```python
from build123d import *

# Parameters (mm, degrees)
BOSS_EXTRUDE1_DEPTH   = 20
BOSS_EXTRUDE1_2_DEPTH = 20
BOSS_EXTRUDE1_3_DEPTH = 20
BOSS_EXTRUDE1_4_DEPTH = 20
SKETCH2_W             = 20
SKETCH2_H             = 20
BOSS_EXTRUDE2_DEPTH   = 20
CUT_EXTRUDE1_DEPTH    = 31
BOSS_EXTRUDE3_DEPTH   = 30
FILLET1_R             = 7
CUT_EXTRUDE2_REACH    = 47.826
SKETCH5_R             = 2.7
CUT_EXTRUDE3_REACH    = 48.5
SKETCH6_R             = 5
FILLET5_R             = 1
FILLET6_R             = 0.75
CUT_EXTRUDE4_DEPTH    = 10


# Some blends are built 0.0001 mm under size
with BuildPart() as part:
    # Sketch1 → Boss-Extrude1 (new body)
    with BuildSketch(Plane(origin=(0, 0, 0), x_dir=(1, 0, 0), z_dir=(0, 1, 0))):
        Polygon((-10, -2.8), (-10, 2.8), (-7.7, 2.8), (-7.7, 5.58), (-7.135634919, 5.58), (-4.28, 2.724365081), (-4.28, -2.724365081), (-7.135634919, -5.58), (-7.7, -5.58), (-7.7, -2.8), align=None)
    extrude(amount=BOSS_EXTRUDE1_DEPTH)



with BuildPart() as body_2:
    # Sketch1 → Boss-Extrude1 2 (new body)
    with BuildSketch(Plane(origin=(0, 0, 0), x_dir=(1, 0, 0), z_dir=(0, 1, 0))):
        Polygon((10, 2.8), (7.7, 2.8), (7.7, 5.58), (7.135634919, 5.58), (4.28, 2.724365081), (4.28, -2.724365081), (7.135634919, -5.58), (7.7, -5.58), (7.7, -2.8), (10, -2.8), align=None)
    extrude(amount=BOSS_EXTRUDE1_2_DEPTH)


with BuildPart() as body_3:
    # Sketch1 → Boss-Extrude1 3 (new body)
    with BuildSketch(Plane(origin=(0, 0, 0), x_dir=(1, 0, 0), z_dir=(0, 1, 0))):
        Polygon((2.8, -10), (-2.8, -10), (-2.8, -7.7), (-5.58, -7.7), (-5.58, -7.135634919), (-2.724365081, -4.28), (2.724365081, -4.28), (5.58, -7.135634919), (5.58, -7.7), (2.8, -7.7), align=None)
    extrude(amount=BOSS_EXTRUDE1_3_DEPTH)


with BuildPart() as body_4:
    # Sketch1 → Boss-Extrude1 4 (new body)
    with BuildSketch(Plane(origin=(0, 0, 0), x_dir=(1, 0, 0), z_dir=(0, 1, 0))):
        Polygon((-2.8, 10), (-2.8, 7.7), (-5.58, 7.7), (-5.58, 7.135634919), (-2.724365081, 4.28), (2.724365081, 4.28), (5.58, 7.135634919), (5.58, 7.7), (2.8, 7.7), (2.8, 10), align=None)
    extrude(amount=BOSS_EXTRUDE1_4_DEPTH)


with BuildPart() as part_1:
    add(part.part)

    add(body_2.part)  # Boss-Extrude2 merges body 2

    add(body_3.part)  # Boss-Extrude2 merges body 3

    add(body_4.part)  # Boss-Extrude2 merges body 4
    # Sketch2 → Boss-Extrude2 (add)
    with BuildSketch(Plane.XZ):
        Rectangle(SKETCH2_W, SKETCH2_H)
    extrude(amount=BOSS_EXTRUDE2_DEPTH)

    # Sketch3 → Cut-Extrude1 (cut, through all)
    with BuildSketch(Plane(origin=(10, 0, 0), x_dir=(0, 0, -1), z_dir=(1, 0, 0))):
        Polygon((10.596673941, -8.137212268), (10.596673941, -38.345549702), (-10.411138478, -38.345549702), (-10.411138478, -2.402671747), align=None)
    extrude(amount=-CUT_EXTRUDE1_DEPTH, mode=Mode.SUBTRACT)

    # Sketch4 → Boss-Extrude3 (add)
    with BuildSketch(Plane.ZY.offset(10)):
        Polygon((10, 0), (-10, 0), (-10, -7.974337104), (10, -2.51490096), align=None)
    extrude(amount=BOSS_EXTRUDE3_DEPTH)

    # Fillet1
    # the kernel refuses this fillet: 7 mm, written as the material it takes off along each edge
    with BuildSketch(Plane(origin=(10, 2.093496024, 26.882318479), x_dir=(0, 0.9647039130954435, -0.26333697054978655), z_dir=(0, -0.26333697054978655, -0.9647039130954435))) as fillet1_piece_1:
        with BuildLine():
            CenterArc((FILLET1_R, -FILLET1_R), FILLET1_R, 90, 90)
            Line((0, -FILLET1_R), (0, 0))
            Line((0, 0), (FILLET1_R, 0))
        make_face()
    extrude(amount=55.731749637, mode=Mode.SUBTRACT)

    # Cut-Extrude2: up to this plane
    cut_extrude2_end = Plane(origin=(-10, -8.137212268, -10.596673941), z_dir=(0, 0.9647039130954435, -0.26333697054978655))
    # Sketch5 → Cut-Extrude2 (cut, up to the surface)
    with BuildSketch(Plane(origin=(0, 0, 0), x_dir=(1, 0, 0), z_dir=(0, 1, 0)), mode=Mode.PRIVATE) as cut_extrude2_sk1:
        with Locations(Location((-28.5, 0, 0), (0, 0, 270))):
            Circle(SKETCH5_R)
    cut_extrude2_tool1 = split(extrude(cut_extrude2_sk1.sketch, amount=-CUT_EXTRUDE2_REACH, mode=Mode.PRIVATE), bisect_by=cut_extrude2_end, keep=Keep.BOTH, mode=Mode.PRIVATE)
    add(cut_extrude2_tool1.solids().sort_by_distance((-28.5, 0, 0))[0], mode=Mode.SUBTRACT)

    # Cut-Extrude3: up to this plane
    cut_extrude3_end = Plane(origin=(-10, -8.137212268, -10.596673941), z_dir=(0, 0.9647039130954435, -0.26333697054978655))
    # Sketch6 → Cut-Extrude3 (cut, up to the surface)
    with BuildSketch(Plane(origin=(0, -1.5, 0), x_dir=(1, 0, 0), z_dir=(0, 1, 0)), mode=Mode.PRIVATE) as cut_extrude3_sk1:
        with Locations(Location((-28.5, 0, 0), (0, 0, 270))):
            Circle(SKETCH6_R)
    cut_extrude3_tool1 = split(extrude(cut_extrude3_sk1.sketch, amount=-CUT_EXTRUDE3_REACH, mode=Mode.PRIVATE), bisect_by=cut_extrude3_end, keep=Keep.BOTH, mode=Mode.PRIVATE)
    add(cut_extrude3_tool1.solids().sort_by_distance((-28.5, -1.5, 0))[0], mode=Mode.SUBTRACT)

    # Fillet5
    fillet5_edges = [part_1.edges().sort_by_distance(p)[0] for p in [
        (-4.28, 0, 0),
        (-5.707817459, 0, 4.152182541),
        (-7.417817459, 0, 5.58),
        (-7.7, 0, 4.19),
        (-8.85, 0, 2.8),
        (-10, 0, 0),
        (-8.85, 0, -2.8),
        (-7.7, 0, -4.19),
        (-5.707817459, 0, -4.152182541),
        (-7.417817459, 0, -5.58),
        (-2.8, 0, -8.85),
        (-4.19, 0, -7.7),
        (-5.58, 0, -7.417817459),
        (-4.152182541, 0, -5.707817459),
        (0, 0, -4.28),
        (4.152182541, 0, -5.707817459),
        (5.58, 0, -7.417817459),
        (4.19, 0, -7.7),
        (2.8, 0, -8.85),
        (8.79791333, 0, -2.8),
        (7.7, 0, -4.19),
        (7.417817459, 0, -5.58),
        (5.707817459, 0, -4.152182541),
        (4.28, 0, 0),
        (5.707817459, 0, 4.152182541),
        (7.417817459, 0, 5.58),
        (8.583774042, 0, 2.8),
        (7.7, 0, 4.19),
        (2.8, 0, 8.85),
        (4.19, 0, 7.7),
        (5.58, 0, 7.417817459),
        (4.152182541, 0, 5.707817459),
        (0, 0, 4.28),
        (-4.152182541, 0, 5.707817459),
        (-5.58, 0, 7.417817459),
        (-4.19, 0, 7.7),
        (-2.8, 0, 8.85),
    ]]
    fillet(fillet5_edges, radius=FILLET5_R)

    # Fillet6
    fillet6_edges = [part_1.edges().sort_by_distance(p)[0] for p in [
        (-28.5, 0, -2.7),
        (-28.5, -6.609478068, -5),
        (-28.5, -1.5, -2.7),
        (-28.5, -1.5, -5),
    ]]
    fillet(fillet6_edges, radius=FILLET6_R - 0.0001)  # a hair under: the kernel refuses the full size

    # Sketch7 → Cut-Extrude4 (cut)
    with BuildSketch(Plane(origin=(0, 20, 0), x_dir=(1, 0, 0), z_dir=(0, 1, 0))):
        Polygon((-7.555562818, 7.211994187), (-2.766940799, 2.423372169), (-2.766940799, -2.697134544), (-7.555562818, -7.485756562), (-13.102778423, -7.485756562), (-13.102778423, 7.211994187), align=None)
    extrude(amount=-CUT_EXTRUDE4_DEPTH, mode=Mode.SUBTRACT)


solid = part_1.part
```
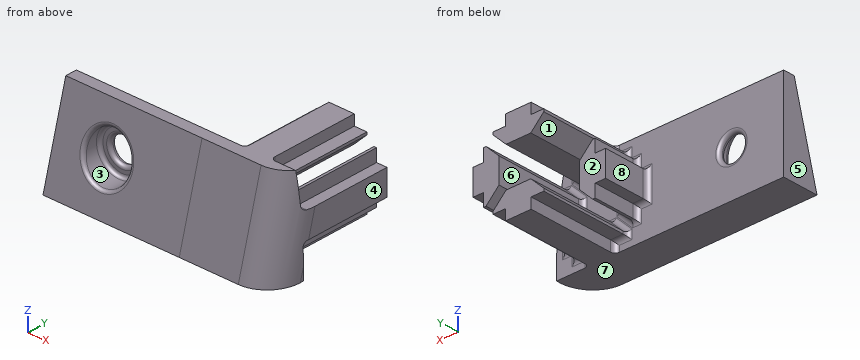
For this review, take the finished solid that the model builds, in its own axes (mm). Face numbers are marked on the shaded views. A direction names the side the tool comes from. Coordinates: 2 decimals unless noted, no trailing zeros. Loops run counter-clockwise (first coordinate to the right, second up) from the corner with the lowest first, then second, coordinate; pieces in that order, holes last. Notation, with made-up numbers: (-4, 70.5) -> (6, 70.5) arc R8 cw to (6, 85.5) -> close; hole circle Ø3 at (75, -35.75). An arc over 180 degrees is marked (long way). Return JSON: item names as keys, results as strings. Group by question number.
(1) Mouldability with a two-part tool opening along Z and no side actions: class the marked faces 6, 7 and 8 as pulls with the +Z half, pulls with the -Z half, needs draft (parallel to the pull), parting line crosses it, or undercut.
(2) Tool access review of the marked faces 1, 2, 3, 4 and 5: name each direction out of +Z, -Z, +X, -X, +Y, -Y from which nothing blocks a thin tool from reaching the whole face with its end or side.
(3) For pin 1 Ø4.5 at (y, z) = (14.5, 0) entering from -X; pin 2 Ø10 at (x, z) = (-25, -3) entering from +Y; pin 3 Ø1.8 at (y, z) = (6.5, 9) entering from -X; pin 4 Ø2 at (x, y) = (-3.5, 14) entering from -Z, all flat-tipped, find the tip position at first contact; note any pin that passes through.
(4) Consider section D-D, the plane x = -13. Give the boundary of the cut face in (y, z).
(5) Consider section C-C, the plane x = -1. Give the boundary of the cut face in (y, z).
(6) To check wall thickness, follow L1, parallel to Z at x = 8, y = 11.5; L2, parallel to X at y = -4.65, z = 0; L3, parallel to X at y = -4.5, z = 0. State the ranges of each line that lie inside material, in increasing order.
(7) Consider section A-A, the plane y = 16.5. Count the separate pieces of the cut face and the enclosed holes in it, plus the area to 3 significant figures.
Results below:
{
 "1": {"face 6": "undercut", "face 7": "pulls with the -Z half", "face 8": "needs draft"},
 "2": {"face 1": "+Y", "face 2": "-X, +Y", "face 3": "-Y", "face 4": "+Z, -Z, +X, +Y, -Y", "face 5": "+Z, -Z, -X, +Y, -Y"},
 "3": {"pin 1": "stops at x = 4.28", "pin 2": "stops at y = 0", "pin 3": "stops at x = -2.8", "pin 4": "stops at z = -10"},
 "4": {"outline": "(-7.97, -10) -> (0, -10) -> (0, 10) -> (-2.51, 10) -> close"},
 "5": {"outline": "(-7.97, -10) -> (20, -10) -> (20, -4.28) -> (1, -4.28) arc R1 cw to (0, -3.28) -> (0, 3.28) arc R1 cw to (1, 4.28) -> (20, 4.28) -> (20, 10) -> (-2.51, 10) -> close"},
 "6": {"L1": "z = -2.8 to 2.8", "L2": "x = -40 to -33.52, -23.48 to 5.78", "L3": "x = -40 to -33.5, -23.5 to 6.09"},
 "7": {"separate pieces": "3", "enclosed holes": "0", "area": "129 mm2"}
}
